```python
from build123d import *

# Parameters (mm, degrees)
BOSS_EXTRUDE1_DEPTH = 69
SKETCH2_R           = 4
CUT_EXTRUDE1_DEPTH  = 11
SKETCH3_R           = 3
CUT_EXTRUDE2_DEPTH  = 10


with BuildPart() as part:
    # Sketch1 → Boss-Extrude1 (new body)
    with BuildSketch(Plane(origin=(0, 0, 0), x_dir=(0, 0, -1), z_dir=(1, 0, 0))):
        Polygon((0, 80.15), (0, 0), (35, 0), (35, 10), (10, 10), (10, 80.15), align=None)
    extrude(amount=BOSS_EXTRUDE1_DEPTH)

    # Sketch2 → Cut-Extrude1 (cut, through all)
    with BuildSketch(Plane(origin=(0, 0, -10), x_dir=(-1, 0, 0), z_dir=(0, 0, -1))):
        with Locations((-34.5, 71.08)):
            Circle(SKETCH2_R)
        with Locations((-34.5, 49.08)):
            Circle(SKETCH2_R)
    extrude(amount=-CUT_EXTRUDE1_DEPTH, mode=Mode.SUBTRACT)

    # Sketch3 → Cut-Extrude2 (cut)
    with BuildSketch(Plane(origin=(0, 10, 0), x_dir=(1, 0, 0), z_dir=(0, 1, 0))):
        with Locations((17, 22.5)):
            Circle(SKETCH3_R)
        with Locations((52, 22.5)):
            Circle(SKETCH3_R)
    extrude(amount=-CUT_EXTRUDE2_DEPTH, mode=Mode.SUBTRACT)


solid = part.part
```
Model file for the job. Use its own axes, mm. A direction names the side the tool comes from. Coordinates: 2 decimals unless noted, no trailing zeros. Order: outer loops, then holes, each group sorted by start corner. A loop starts at its lowest first (then second) coordinate and runs counter-clockwise, first axis right, second up. Notation, with made-up numbers: (41.5, 69.5) -> (80.5, 69.5) arc R21 cw to (80.5, 87.5) -> close; hole circle Ø3 at (33.5, 76). An arc over 180 degrees is marked (long way). Answer as a JSON object with one key per item and string values. Group by question number.
1) Which spindle directions (+Z, -Z, +X, -X, +Y, -Y) get a long thin tool onto all of the face, cutting with end or side? Do faces 4 (the face through (34, 0, -17)), 5 (the face through (34, 44.6, -10)). Say none if no direction does.
2) Cut at A-A, the plane y = 71.08. Write the cut outline in (x, z).
3) Pull direction X, two halves, no side cores. Call faces 1 (the face through (14.6, 5.1, -20.7)), 2 (the face through (69, 32, -9)), 3 (the face through (34, 80.15, -5)): +X half, -X half, draft (parallel to the pull), parting line (faces both ways), or undercut.
4) Cut at D-D, the plane x = 17. Write the cut outline in (y, z), then the cut area to 4 significant figures.
5) Cut at C-C, the plane x = 34.5. Write the cut outline in (y, z).
6) Flat gauge pins, fed straight in: pin 1 (20.5 mm diameter, centred on x = 30.5, y = 39, fed in from -Z); pin 2 (1.5 mm diameter, centred on y = 33.5, z = -6.5, fed in from -X); pin 3 (1 mm diameter, centred on x = 9, z = -16.5, fed in from +Y). Where does each tip first touch, or does it go through?
7) Drill centre lines: L1, parallel to Y at x = 34.5, z = -6.5; L2, parallel to Z at x = 52, y = 3; L3, parallel to Z at x = 17.5, y = 77.5. Where is each one in solid material? Low to high.
8) Cut at B-B, the plane z = -22.5. Write the cut outline in (x, y).
Check values:
{
 "1": {"face 4": "+Z, -Z, +X, -X, -Y", "face 5": "-Z, +X, -X, +Y"},
 "2": {"outline": "(0, -10) -> (30.5, -10) -> (30.5, 0) -> (0, 0) -> close; (38.5, -10) -> (69, -10) -> (69, 0) -> (38.5, 0) -> close"},
 "3": {"face 1": "undercut", "face 2": "+X half", "face 3": "draft"},
 "4": {"outline": "(0, -35) -> (10, -35) -> (10, -25.5) -> (0, -25.5) -> close; (0, -19.5) -> (10, -19.5) -> (10, -10) -> (80.15, -10) -> (80.15, 0) -> (0, 0) -> close", "area": "991.5 mm²"},
 "5": {"outline": "(0, -35) -> (10, -35) -> (10, -10) -> (45.08, -10) -> (45.08, 0) -> (0, 0) -> close; (53.08, -10) -> (67.08, -10) -> (67.08, 0) -> (53.08, 0) -> close; (75.08, -10) -> (80.15, -10) -> (80.15, 0) -> (75.08, 0) -> close"},
 "6": {"pin 1": "stops at z = -10", "pin 2": "stops at x = 0", "pin 3": "stops at y = 10"},
 "7": {"L1": "y = 0 to 45.08, 53.08 to 67.08, 75.08 to 80.15", "L2": "z = -35 to -25.5, -19.5 to 0", "L3": "z = -10 to 0"},
 "8": {"outline": "(0, 0) -> (14, 0) -> (14, 10) -> (0, 10) -> close; (20, 0) -> (49, 0) -> (49, 10) -> (20, 10) -> close; (55, 0) -> (69, 0) -> (69, 10) -> (55, 10) -> close"}
}
